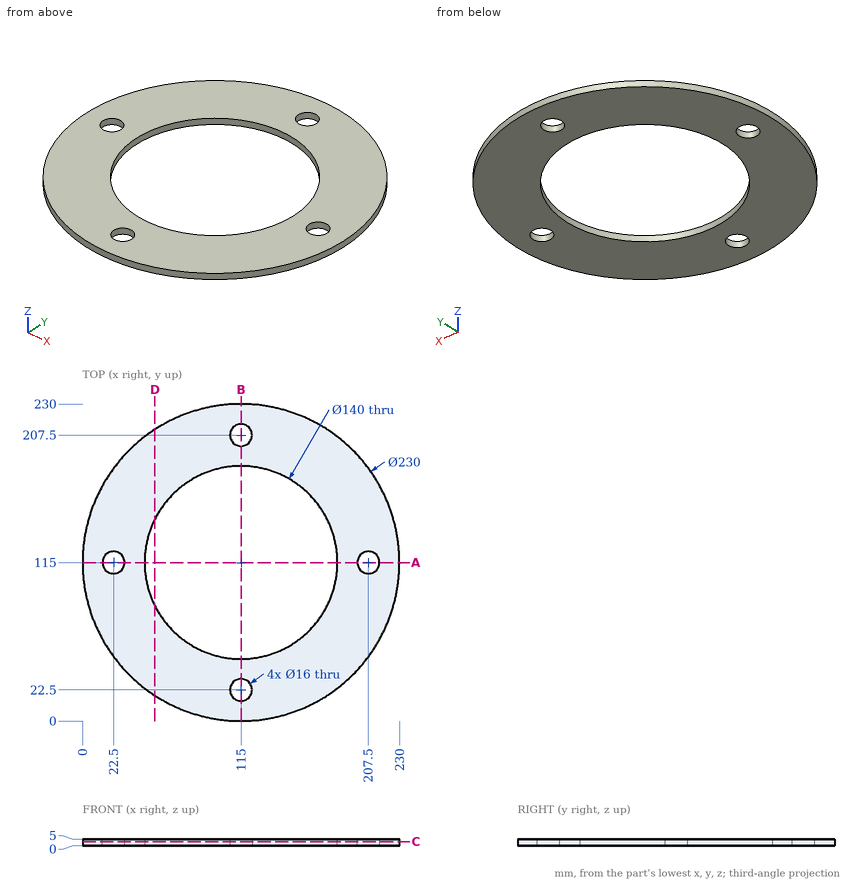
Answer from the drawing. Dimensions are ordinates in mm from the lowest x, y and z of the part. Coordinates: 2 decimals unless noted, no trailing zeros. Loops run counter-clockwise (first coordinate to the right, second up) from the corner with the lowest first, then second, coordinate; pieces in that order, holes last.
1) Section A-A (y = 115) is taken. Give the vertices of the cut face in (x, z), plus the area to 3 significant figures.
Results:
outline: (0, 0) - (14.5, 0) - (14.5, 5) - (0, 5) - close; (30.5, 0) - (45, 0) - (45, 5) - (30.5, 5) - close; (185, 0) - (199.5, 0) - (199.5, 5) - (185, 5) - close; (215.5, 0) - (230, 0) - (230, 5) - (215.5, 5) - close
area: 290 mm2
2) Consider probe 1 along Y at (x, z) = (115, 2.1); probe 2 along Y at (x, z) = (22.5, 4); probe 3 along Y at (x, z) = (213.5, 4.2). Determine where each line is inside the solid, lowest interval first.
Results:
probe 1: y = 0 to 14.5, 30.5 to 45, 185 to 199.5, 215.5 to 230
probe 2: y = 46.67 to 107, 123 to 183.33
probe 3: y = 55.65 to 109.71, 120.29 to 174.35
3) Section C-C (z = 3.05) is taken. Give the vertices of the cut face in (x, y).
Results:
outline: circle Ø230 at (115, 115); hole circle Ø16 at (22.5, 115); hole circle Ø140 at (115, 115); hole circle Ø16 at (115, 22.5); hole circle Ø16 at (115, 207.5); hole circle Ø16 at (207.5, 115)
4) Section D-D (x = 52.5) is taken. Give the vertices of the cut face in (y, z), plus the area to 3 significant figures.
Results:
outline: (18.47, 0) - (83.48, 0) - (83.48, 5) - (18.47, 5) - close; (146.52, 0) - (211.53, 0) - (211.53, 5) - (146.52, 5) - close
area: 650 mm2
5) Flat-ended cylindrical pins translate along their axes: pin 1 (1.5 mm diameter, centred on y = 130.5, z = 1.5, fed in from +X); pin 2 (1 mm diameter, centred on x = 120.5, z = 2, fed in from +Y). Find the tip coordinate at first contact, or state that the pin passes through.
Results:
pin 1: stops at x = 229.05
pin 2: stops at y = 229.89
